from build123d import *

# Parameters (mm, degrees)
SKETCH3_R           = 1.7
BOSS_EXTRUDE4_DEPTH = 3
CUT_EXTRUDE3_REACH  = 5
SKETCH4_R           = 1.2


with BuildPart() as part:
    # Sketch1 → Revolve1 (revolve)
    with BuildSketch(Plane.XY):
        Polygon((11.7, 0), (0, 0), (0, 3), (13.3, 3), (13.3, -16), (11.7, -16), align=None)
        Polygon((16.3, -11.9), (13.3, -11.9), (13.3, -16), (16.3, -14.9), align=None)
    revolve(axis=Axis((0, -272.323852837, 0), (0, 1, 0)))

    # Sketch3 → Boss-Extrude4 (add)
    with BuildSketch(Plane(origin=(0, -11.9, 0), x_dir=(1, 0, 0), z_dir=(0, 1, 0))):
        with BuildLine():
            ThreePointArc((-20.029124088, 5.699925595), (-25.7, 0), (-20.029124088, -5.699925595))
            ThreePointArc((-20.029124088, -5.699925595), (-16.315754318, -6.635428811), (-13.462592593, -9.189591976))
            ThreePointArc((-13.462592593, -9.189591976), (-16.3, 0), (-13.462592593, 9.189591976))
            ThreePointArc((-13.462592593, 9.189591976), (-16.315754318, 6.635428811), (-20.029124088, 5.699925595))
        make_face()
        with Locations((-20, 0)):
            Circle(SKETCH3_R, mode=Mode.SUBTRACT)
        with BuildLine():
            ThreePointArc((13.462592593, -9.189591976), (16.3, 0), (13.462592593, 9.189591976))
            ThreePointArc((13.462592593, 9.189591976), (16.315754318, 6.635428811), (20.029124088, 5.699925595))
            ThreePointArc((20.029124088, 5.699925595), (25.7, 0), (20.029124088, -5.699925595))
            ThreePointArc((20.029124088, -5.699925595), (16.315754318, -6.635428811), (13.462592593, -9.189591976))
        make_face()
        with Locations((20, 0)):
            Circle(SKETCH3_R, mode=Mode.SUBTRACT)
    extrude(amount=-BOSS_EXTRUDE4_DEPTH)

    # Sketch4 → Cut-Extrude3 (cut, up to next)
    with BuildSketch(Plane(origin=(0, 0, 0), x_dir=(1, 0, 0), z_dir=(0, 1, 0)), mode=Mode.PRIVATE) as cut_extrude3_sk1:
        with Locations((7.75, 0)):
            Circle(SKETCH4_R)
    cut_extrude3_tool1 = extrude(cut_extrude3_sk1.sketch, amount=CUT_EXTRUDE3_REACH, mode=Mode.PRIVATE) & part.part
    add(cut_extrude3_tool1.solids().sort_by_distance((7.75, 0, 0))[0], mode=Mode.SUBTRACT)
    # Sketch4 → Cut-Extrude3 (cut, up to next)
    with BuildSketch(Plane(origin=(0, 0, 0), x_dir=(1, 0, 0), z_dir=(0, 1, 0)), mode=Mode.PRIVATE) as cut_extrude3_sk2:
        with Locations((-7.75, 0)):
            Circle(SKETCH4_R)
    cut_extrude3_tool2 = extrude(cut_extrude3_sk2.sketch, amount=CUT_EXTRUDE3_REACH, mode=Mode.PRIVATE) & part.part
    add(cut_extrude3_tool2.solids().sort_by_distance((-7.75, 0, 0))[0], mode=Mode.SUBTRACT)


solid = part.part
The listing builds one solid part. Answer for the finished solid, in the listing's coordinates (mm). A direction names the side the tool comes from. Round coordinates to 2 decimals unless told otherwise and drop trailing zeros. Write each loop counter-clockwise with the first axis right and the second up, starting at its lowest first coordinate (ties: lowest second). Pieces come first, ordered by that corner, then holes. Notation, with made-up numbers: M -17,-6 L 40,-6 A30 cw 40,32 Z; hole C -1.5,-26.75 d10. An arc over 180 degrees is marked long. Write each question's results on one line, items separated by ' | '. Start each with the question number.
Item 1: Given pin 1 Ø18.5 at (x, z) = (0, 0) entering from -Y; pin 2 Ø6 at (x, z) = (20.5, 0) entering from -Y; pin 3 Ø8 at (y, z) = (-13.5, 7) entering from -X; pin 4 Ø6 at (x, y) = (-19.5, -7) entering from +Z, each flat-ended and moving along its own axis, determine where each tip first touches the part or whether it passes through.
Item 2: Straight lines are drawn through the part: probe 1 along X at (y, z) = (2.05, 0); probe 2 along X at (y, z) = (-13.5, 0); probe 3 along X at (y, z) = (-5.5, 0). For each, find the intervals that lie inside material, in ascending order.
Item 3: Which of the six approach directions +Z, -Z, +X, -X, +Y, -Y give full straight-line access (tool end or side, diameter ignored) to faces 1 (the cylindrical face through (16.36, -13.38, 6.61)), 2 (the cylindrical face through (6.14, -4.55, 11.8)), 3 (the flat face through (0, 0, 0))?
Item 4: Find section B-B on z = 0. Give the number of separate pieces and of enclosed holes in the cut face, and give its area (3 significant figures).
Item 5: Find section C-C on x = 0. Write down the section's boundary in (y, z), and give its area (3 significant figures).
Item 6: Find section A-A on y = -14.25. Write down the section's boundary in (x, z), and give its area (3 significant figures).
Item 7: Find section D-D on y = -7. Write down the section's boundary in (x, z).
Item 8: The mould has two halves that part along Z. Classify faces 4 (the cylindrical face through (-0.2, -13.4, 16.3)), 5 (the cylindrical face through (-2.54, -7.89, 11.42)), 6 (the flat face through (8, -11.9, -11)), 7 (the cylindrical face through (-8.95, 1.48, -0.05)): +Z half, -Z half, draft (parallel to the pull), parting line (faces both ways), or undercut.
Answer block:
1) pin 1: stops at y = 0 | pin 2: stops at y = -14.9 | pin 3: stops at x = -24.85 | pin 4: passes through
2) probe 1: x = -13.3 to -8.95, -6.55 to 6.55, 8.95 to 13.3 | probe 2: x = -25.7 to -21.7, -18.3 to -11.7, 11.7 to 18.3, 21.7 to 25.7 | probe 3: x = -13.3 to -11.7, 11.7 to 13.3
3) face 1: +Z, +X, +Y, -Y | face 2: +Y | face 3: -Y
4) separate pieces: 5 | enclosed holes: 0 | area: 174 mm²
5) outline: M -16,-13.3 L -14.9,-16.3 L -11.9,-16.3 L -11.9,-13.3 L 3,-13.3 L 3,13.3 L -11.9,13.3 L -11.9,16.3 L -14.9,16.3 L -16,13.3 L -16,11.7 L 0,11.7 L 0,-11.7 L -16,-11.7 Z | area: 152 mm²
6) outline: M -20.03,-5.7 A8 cw -13.46,-9.19 A16.3 ccw 13.46,-9.19 A8 cw 20.03,-5.7 A5.7 ccw 20.03,5.7 A8 cw 13.46,9.19 A16.3 ccw -13.46,9.19 A8 cw -20.03,5.7 A5.7 ccw Z; hole C -20,0 d3.4; hole C 0,0 d23.4; hole C 20,0 d3.4 | area: 594 mm²
7) outline: C 0,0 d26.6; hole C 0,0 d23.4
8) face 4: +Z half | face 5: undercut | face 6: draft | face 7: undercut
